```python
from build123d import *

# Parameters (mm, degrees)
SKETCH1_R                      = 4.445
BOSS_EXTRUDE1_DEPTH            = 3.175
SKETCH2_R                      = 3.175
BOSS_EXTRUDE2_DEPTH            = 16.4338
BOSS_EXTRUDE3_START            = 12.7
SKETCH3_R                      = 3.175
BOSS_EXTRUDE3_DEPTH            = 12.7
CHAMFER1_SIZE                  = 6.35
CHAMFER1_SIZE2                 = 3.165993211
SKETCH4_R                      = 2.1828125
CUT_EXTRUDE1_DEPTH             = 6.35
SKETCH5_R                      = 1.7859375
CUT_EXTRUDE2_DEPTH             = 1.905
CUT_EXTRUDE5_REACH             = 22.592
CUT_EXTRUDE5_END_RADIUS        = 3.175
SKETCH7_R                      = 1.4224
CUT_EXTRUDE5_DIRECTION_2_DEPTH = 21.591772324


with BuildPart() as part:
    # Sketch1 → Boss-Extrude1 (new body)
    with BuildSketch(Plane(origin=(0, 0, 0), x_dir=(0, 0, -1), z_dir=(1, 0, 0))):
        Circle(SKETCH1_R)
    extrude(amount=BOSS_EXTRUDE1_DEPTH)

    # Sketch2 → Boss-Extrude2 (add)
    with BuildSketch(Plane(origin=(3.175, 0, 0), x_dir=(0, 0, -1), z_dir=(1, 0, 0))):
        Circle(SKETCH2_R)
    extrude(amount=BOSS_EXTRUDE2_DEPTH)

    # Sketch3 → Boss-Extrude3 (add)
    with BuildSketch(Plane.ZY.offset(BOSS_EXTRUDE3_START)):
        with Locations(Location((0, 0, 0), (0, 0, 180))):
            Circle(SKETCH3_R)
    extrude(amount=-BOSS_EXTRUDE3_DEPTH)

    # Chamfer1
    chamfer1_edges = [part.edges().sort_by_distance(p)[0] for p in [
        (19.6088, 0, 3.175),
    ]]
    chamfer1_side = [part.faces().sort_by_distance(p)[0] for p in [
        (11.3919, 0, 3.175),
    ]]
    chamfer(chamfer1_edges, length=CHAMFER1_SIZE, length2=CHAMFER1_SIZE2, reference=chamfer1_side[0])

    # Sketch4 → Cut-Extrude1 (cut)
    with BuildSketch(Plane.ZY.offset(12.7)):
        Circle(SKETCH4_R)
    extrude(amount=-CUT_EXTRUDE1_DEPTH, mode=Mode.SUBTRACT)

    # Sketch5 → Cut-Extrude2 (cut)
    with BuildSketch(Plane.ZY.offset(6.35)):
        Circle(SKETCH5_R)
    extrude(amount=-CUT_EXTRUDE2_DEPTH, mode=Mode.SUBTRACT)

    # Cut-Extrude5: up to this cylinder (the profile starts inside it)
    cut_extrude5_end = Plane(origin=(-9.525, 0, 0), z_dir=(1, 0, 0)) * Cylinder(CUT_EXTRUDE5_END_RADIUS, 52.534, mode=Mode.PRIVATE)
    # Sketch7 → Cut-Extrude5 (cut, up to the surface)
    with BuildSketch(Plane.XY, mode=Mode.PRIVATE) as cut_extrude5_sk1:
        with Locations(Location((-9.525, 0, 0), (0, 0, 180))):
            Circle(SKETCH7_R)
    cut_extrude5_tool1 = extrude(cut_extrude5_sk1.sketch, amount=CUT_EXTRUDE5_REACH, mode=Mode.PRIVATE) & cut_extrude5_end
    add(cut_extrude5_tool1.solids().sort_by_distance((-9.525, 0, 0))[0], mode=Mode.SUBTRACT)

    # Sketch7 → Cut-Extrude5 direction 2 (cut)
    with BuildSketch(Plane.XY):
        with Locations(Location((-9.525, 0, 0), (0, 0, 180))):
            Circle(SKETCH7_R)
    extrude(amount=-CUT_EXTRUDE5_DIRECTION_2_DEPTH, mode=Mode.SUBTRACT)


solid = part.part
```
Check sheet for the modelled part. Datum: model origin and axes. Units: mm. A direction names the side the tool comes from. Round coordinates to 2 decimals unless told otherwise and drop trailing zeros. Loops run counter-clockwise (first coordinate to the right, second up) from the corner with the lowest first, then second, coordinate; pieces in that order, holes last. Notation, with made-up numbers: (8.5, -18.75) - (64.5, -18.75) arc R19 cw to (64.5, 3.25) - close; hole circle Ø11 at (19, -21.5). An arc over 180 degrees is marked (long way). Answer as a JSON object with one key per item and string values. Group by question number.
Q1. Gauge pin test, flat ends, axial feed: P1, Ø2, axis at x = 14.5, y = 0, coming from the -Z side; P2, Ø2.5, axis at y = 1, z = 1, coming from the +X side; P3, Ø4.5, axis at x = -9.525, y = 0, coming from the -Z side (3 decimals); P4, Ø2.5, axis at x = -9.525, y = 0, coming from the -Z side. Record the tip position at first contact, or that the pin passes through.
Q2. Mould release check, pull along Z, two halves, no side actions. Record for faces 3 (the face through (8.15, -3.1, 0.69)), 4 (the face through (-9.569, 2.164, -0.284)), 5 (the face through (-6.35, 0, -2)), 6 (the face through (3.175, -3, -2)): released by +Z, released by -Z, zero draft, split by the parting line, or undercut.
Q3. Scan lines: line 1 along Y through (x, z) = (-10.25, 0) (3 decimals); line 2 along Y through (x, z) = (-4.75, 0) (3 decimals); line 3 along X through (y, z) = (3, -3) (3 decimals). Record each from-to range of solid material in increasing order. Write a range as [from, to].
Q4. Set-up check for faces 1 (the face through (-12.7, -2.2, 0.8)), 2 (the face through (-5.411, 0.079, -1.784)): record each of +Z, -Z, +X, -X, +Y, -Y from which the full face is reachable in a straight line by a thin tool's end or side.
Q5. Sectioned sample at A-A, the plane x = -8.5. Enter the section's corners in (y, z) (3 decimals).
Q6. Sectioned sample at D-D, the plane x = 17.5. Enter the section's corners in (y, z), plus the area to 3 significant figures.
Q7. Sectioned sample at C-C, the plane x = 6.5. Enter the section's corners in (y, z) (3 decimals), plus the area to 3 significant figures.
Q8. Sectioned sample at B-B, the plane z = 4. Enter the section's corners in (x, y) (3 decimals), plus the area to 3 significant figures.
Solution:
{
 "1": {"P1": "stops at z = -3.05", "P2": "stops at x = 19.3", "P3": "stops at z = -3.175", "P4": "passes through"},
 "2": {"face 3": "split by the parting line", "face 4": "undercut", "face 5": "undercut", "face 6": "zero draft"},
 "3": {"line 1": "y = [-3.175, -2.183], [2.183, 3.175]", "line 2": "y = [-3.175, -1.786], [1.786, 3.175]", "line 3": "x = [0, 3.175]"},
 "4": {"face 1": "+Z, -Z, -X, +Y, -Y", "face 2": "-X"},
 "5": {"outline": "(-0.986, -3.018) - (-0.986, -1.947) arc R2.183 cw to (-0.986, 1.947) - (-0.986, 3.018) arc R3.175 ccw to start; (0.986, -3.018) arc R3.175 ccw to (0.986, 3.018) - (0.986, 1.947) arc R2.183 cw to (0.986, -1.947) - close"},
 "6": {"outline": "circle Ø2.12 at (0, 0)", "area": "3.53 mm²"},
 "7": {"outline": "circle Ø6.35 at (0, 0)", "area": "31.7 mm²"},
 "8": {"outline": "(0, -1.939) - (3.175, -1.939) - (3.175, 1.939) - (0, 1.939) - close", "area": "12.3 mm²"}
}
